from build123d import *

# Parameters (mm, degrees)
IZIM1_R                     = 117.5
IZIM1_R_2                   = 32.5
IZIM1_R_3                   = 5
Y_KSEKLIK_EKSTR_ZYON1_DEPTH = 2
IZIM1_2_R                   = 35.5
IZIM1_2_R_2                 = 32.5
EKSTR_ZYON_NCE1_DEPTH       = 40
IZIM2_R                     = 10
IZIM2_R_2                   = 8
EKSTR_ZYON_NCE2_DEPTH       = 10


with BuildPart() as part:
    # Çizim1 → Yükseklik-Ekstrüzyon1 (new body)
    with BuildSketch(Plane(origin=(0, 0, 0), x_dir=(1, 0, 0), z_dir=(0, 1, 0))):
        Circle(IZIM1_R)
        with Locations((0, 70)):
            Circle(IZIM1_R_2, mode=Mode.SUBTRACT)
        with Locations((50, 0)):
            Circle(IZIM1_R_2, mode=Mode.SUBTRACT)
        with Locations((0, -70)):
            Circle(IZIM1_R_2, mode=Mode.SUBTRACT)
        with Locations((-50, 0)):
            Circle(IZIM1_R_2, mode=Mode.SUBTRACT)
        Circle(IZIM1_R_3, mode=Mode.SUBTRACT)
    extrude(amount=Y_KSEKLIK_EKSTR_ZYON1_DEPTH)

    # Çizim1<2> → Ekstrüzyon-İnce1 (add)
    with BuildSketch(Plane(origin=(0, 0, 0), x_dir=(1, 0, 0), z_dir=(0, 1, 0))):
        with Locations((0, 70)):
            Circle(IZIM1_2_R)
        with Locations((0, 70)):
            Circle(IZIM1_2_R_2, mode=Mode.SUBTRACT)
        with Locations((50, 0)):
            Circle(IZIM1_2_R)
        with Locations((50, 0)):
            Circle(IZIM1_2_R_2, mode=Mode.SUBTRACT)
        with Locations((0, -70)):
            Circle(IZIM1_2_R)
        with Locations((0, -70)):
            Circle(IZIM1_2_R_2, mode=Mode.SUBTRACT)
        with Locations((-50, 0)):
            Circle(IZIM1_2_R)
        with Locations((-50, 0)):
            Circle(IZIM1_2_R_2, mode=Mode.SUBTRACT)
    extrude(amount=EKSTR_ZYON_NCE1_DEPTH)

    # Çizim2 → Ekstrüzyon-İnce2 (add)
    with BuildSketch(Plane(origin=(0, 2, 0), x_dir=(1, 0, 0), z_dir=(0, 1, 0))):
        with Locations((52, -52)):
            Circle(IZIM2_R)
        with Locations((52, -52)):
            Circle(IZIM2_R_2, mode=Mode.SUBTRACT)
        with Locations((-52, -52)):
            Circle(IZIM2_R)
        with Locations((-52, -52)):
            Circle(IZIM2_R_2, mode=Mode.SUBTRACT)
        with Locations((-52, 52)):
            Circle(IZIM2_R)
        with Locations((-52, 52)):
            Circle(IZIM2_R_2, mode=Mode.SUBTRACT)
        with Locations((52, 52)):
            Circle(IZIM2_R)
        with Locations((52, 52)):
            Circle(IZIM2_R_2, mode=Mode.SUBTRACT)
    extrude(amount=EKSTR_ZYON_NCE2_DEPTH)


solid = part.part
For this review, take the finished solid that the model builds, in its own axes (mm). A direction names the side the tool comes from. Round coordinates to 2 decimals unless told otherwise and drop trailing zeros. Loops run counter-clockwise (first coordinate to the right, second up) from the corner with the lowest first, then second, coordinate; pieces in that order, holes last. Notation, with made-up numbers: (21, -24.75) - (38, -24.75) arc R13 ccw to (38, -1.75) - close; hole circle Ø5 at (6.25, -27.75). An arc over 180 degrees is marked (long way). Answer as CSV lines item,"result".
(1) Consider section A-A on y = 27. Give the boundary of the cut face in (x, z), then the cut area to 3 significant figures.
Checked values:
outline,"circle Ø71 at (-50, 0); circle Ø71 at (0, -70); circle Ø71 at (0, 70); circle Ø71 at (50, 0); hole circle Ø65 at (-50, 0); hole circle Ø65 at (0, -70); hole circle Ø65 at (0, 70); hole circle Ø65 at (50, 0)"
area,"2,560 mm2"
(2) Wall thickness on line 1 (X direction, y = 25.5, z = 0); line 2 (Z direction, x = 52, y = 4); line 3 (X direction, y = 5, z = -52): over which ranges is each line inside the solid? List them lowest first.
Checked values:
line 1,"x = -85.5 to -82.5, -17.5 to -14.5, 14.5 to 17.5, 82.5 to 85.5"
line 2,"z = -62 to -60, -44 to -42, -35.44 to -32.44, 32.44 to 35.44, 42 to 44, 60 to 62"
line 3,"x = -62 to -60, -44 to -42, -30.6 to -27.06, 27.06 to 30.6, 42 to 44, 60 to 62"
(3) Tool access review of faces 5 (the face through (-52, 12, -60.2)), 6 (the face through (-7.696, 20.734, 104.656)), 7 (the face through (-52, 12, 43.8)), 8 (the face through (-82.47, 19.72, -1.43)): name each direction out of +Z, -Z, +X, -X, +Y, -Y from which nothing blocks a thin tool from reaching the whole face with its end or side.
Checked values:
face 5,"-Z, -X, +Y"
face 6,"+Y"
face 7,"+Z, -X, +Y"
face 8,"+Y, -Y"
(4) Consider section D-D on x = 52. Give the boundary of the cut face in (y, z).
Checked values:
outline,"(0, -105.37) - (2, -105.37) - (2, -62) - (12, -62) - (12, -60) - (2, -60) - (2, -44) - (12, -44) - (12, -42) - (2, -42) - (2, -35.44) - (40, -35.44) - (40, -32.44) - (0, -32.44) - close; (0, 32.44) - (40, 32.44) - (40, 35.44) - (2, 35.44) - (2, 42) - (12, 42) - (12, 44) - (2, 44) - (2, 60) - (12, 60) - (12, 62) - (2, 62) - (2, 105.37) - (0, 105.37) - close"
(5) Mouldability with a two-part tool opening along X and no side actions: class faces 1 (the face through (-15.3, 1, -116.5)), 2 (the face through (46.1, 6.9, 46.6)), 3 (the face through (66, 40, 29)), 4 (the face through (-4.6, 20.7, -105.2)) as +X half, -X half, draft (parallel to the pull), parting line (faces both ways), or undercut.
Checked values:
face 1,"parting line"
face 2,"undercut"
face 3,"draft"
face 4,"undercut"
(6) Consider section B-B on y = 8. Give the number of separate pieces and of enclosed holes in the cut face, then the cut area to 3 significant figures.
Checked values:
separate pieces,"8"
enclosed holes,"8"
area,"3,020 mm2"
(7) Insertion check: P1, Ø17.5, axis at x = -49.5, z = 50.5, coming from the +Y side; P2, Ø5, axis at y = 21, z = -26, coming from the +X side; P3, Ø10, axis at y = 32.5, z = -21, coming from the +X side. Each pin has a flat end and moves straight along its axis. Give the tip position at first contact, or say it passes through.
Checked values:
P1,"stops at y = 12"
P2,"stops at x = 76.61"
P3,"stops at x = 81.69"
(8) Consider section C-C on z = 0. Give the boundary of the cut face in (x, y), then the cut area to 3 significant figures.
Checked values:
outline,"(-117.5, 0) - (-82.5, 0) - (-82.5, 40) - (-85.5, 40) - (-85.5, 2) - (-117.5, 2) - close; (-17.5, 0) - (-5, 0) - (-5, 2) - (-14.5, 2) - (-14.5, 40) - (-17.5, 40) - close; (5, 0) - (17.5, 0) - (17.5, 40) - (14.5, 40) - (14.5, 2) - (5, 2) - close; (82.5, 0) - (117.5, 0) - (117.5, 2) - (85.5, 2) - (85.5, 40) - (82.5, 40) - close"
area,"646 mm2"
